```python
from build123d import *

# Parameters (mm, degrees)
ESQUISSE1_R        = 5
ESQUISSE1_R_2      = 1.5
ESQUISSE1_W        = 15
ESQUISSE1_H        = 6
BOSS_EXTRU_1_DEPTH = 6


with BuildPart() as part:
    # Esquisse1 → Boss.-Extru.1 (new body)
    with BuildSketch(Plane.XY):
        Polygon((0, 0), (450, 0), (450, 6), (444, 6), (444, 36), (450, 36), (450, 58.666666667), (444, 58.666666667), (444, 88.666666667), (450, 88.666666667), (450, 111.333333333), (444, 111.333333333), (444, 141.333333333), (450, 141.333333333), (450, 164), (444, 164), (444, 194), (450, 194), (450, 200), (425, 200), (425, 194), (385, 194), (385, 200), (365, 200), (365, 194), (325, 194), (325, 200), (305, 200), (305, 194), (265, 194), (265, 200), (245, 200), (245, 194), (205, 194), (205, 200), (185, 200), (185, 194), (145, 194), (145, 200), (125, 200), (125, 194), (85, 194), (85, 200), (65, 200), (65, 194), (25, 194), (25, 200), (0, 200), (0, 194), (6, 194), (6, 164), (0, 164), (0, 141.333333333), (6, 141.333333333), (6, 111.333333333), (0, 111.333333333), (0, 88.666666667), (6, 88.666666667), (6, 58.666666667), (0, 58.666666667), (0, 36), (6, 36), (6, 6), (0, 6), align=None)
        with Locations((225, 100)):
            Circle(ESQUISSE1_R, mode=Mode.SUBTRACT)
        with Locations((16.25, 124.5)):
            Circle(ESQUISSE1_R_2, mode=Mode.SUBTRACT)
        with Locations((53.75, 124.5)):
            Circle(ESQUISSE1_R_2, mode=Mode.SUBTRACT)
        with Locations(Location((53.75, 75.5, 0), (0, 0, 180))):
            Circle(ESQUISSE1_R_2, mode=Mode.SUBTRACT)
        with Locations(Location((16.25, 75.5, 0), (0, 0, 180))):
            Circle(ESQUISSE1_R_2, mode=Mode.SUBTRACT)
        with Locations((137.5, 24.5)):
            Rectangle(ESQUISSE1_W, ESQUISSE1_H, mode=Mode.SUBTRACT)
        with Locations((102.5, 175.5)):
            Rectangle(ESQUISSE1_W, ESQUISSE1_H, mode=Mode.SUBTRACT)
        with Locations((137.5, 175.5)):
            Rectangle(ESQUISSE1_W, ESQUISSE1_H, mode=Mode.SUBTRACT)
        with Locations((102.5, 24.5)):
            Rectangle(ESQUISSE1_W, ESQUISSE1_H, mode=Mode.SUBTRACT)
    extrude(amount=BOSS_EXTRU_1_DEPTH)


solid = part.part
```
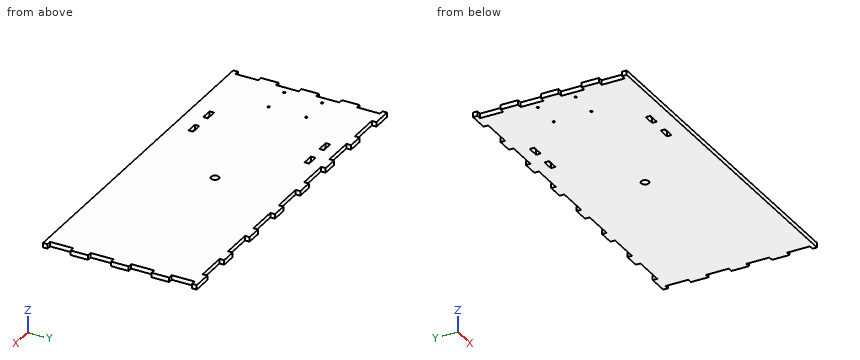
Check sheet for the modelled part. Datum: model origin and axes. Units: mm. Round coordinates to 2 decimals unless told otherwise and drop trailing zeros. Put each result on its own line as item: value.
(1) Material ranges on line 1 (X direction, y = 124.5, z = 3.65); line 2 (Y direction, x = 16.25, z = 2.4); line 3 (Y direction, x = 53.75, z = 3.15), recorded low to high.
Values found:
line 1: x = 6 to 14.75, 17.75 to 52.25, 55.25 to 444
line 2: y = 0 to 74, 77 to 123, 126 to 200
line 3: y = 0 to 74, 77 to 123, 126 to 194
(2) Sectioned sample at A-A (z = 2.05). Count the separate pieces of the cut face and the enclosed holes in it, plus the area to 3 significant figures.
Values found:
separate pieces: 1
enclosed holes: 9
area: 86,400 mm^2
(3) Go/stop test with a flat-tipped pin: pin 1 Ø3 at (y, z) = (67.5, 2.5) entering from +X. Record where the tip stops, or that it passes through.
Values found:
pin 1: stops at x = 444
